Here's the drawing with two shaded views (mm, measured from the low corner). I have some questions. A direction names the side the tool comes from. Round coordinates to 2 decimals unless told otherwise and drop trailing zeros. Loops run counter-clockwise (first coordinate to the right, second up) from the corner with the lowest first, then second, coordinate; pieces in that order, holes last. Notation, with made-up numbers: (37.25, -3) -> (53.25, -3) arc R33 ccw to (53.25, 26) -> close; hole circle Ø7 at (53, -7). An arc over 180 degrees is marked (long way). Write item = value, one per line.
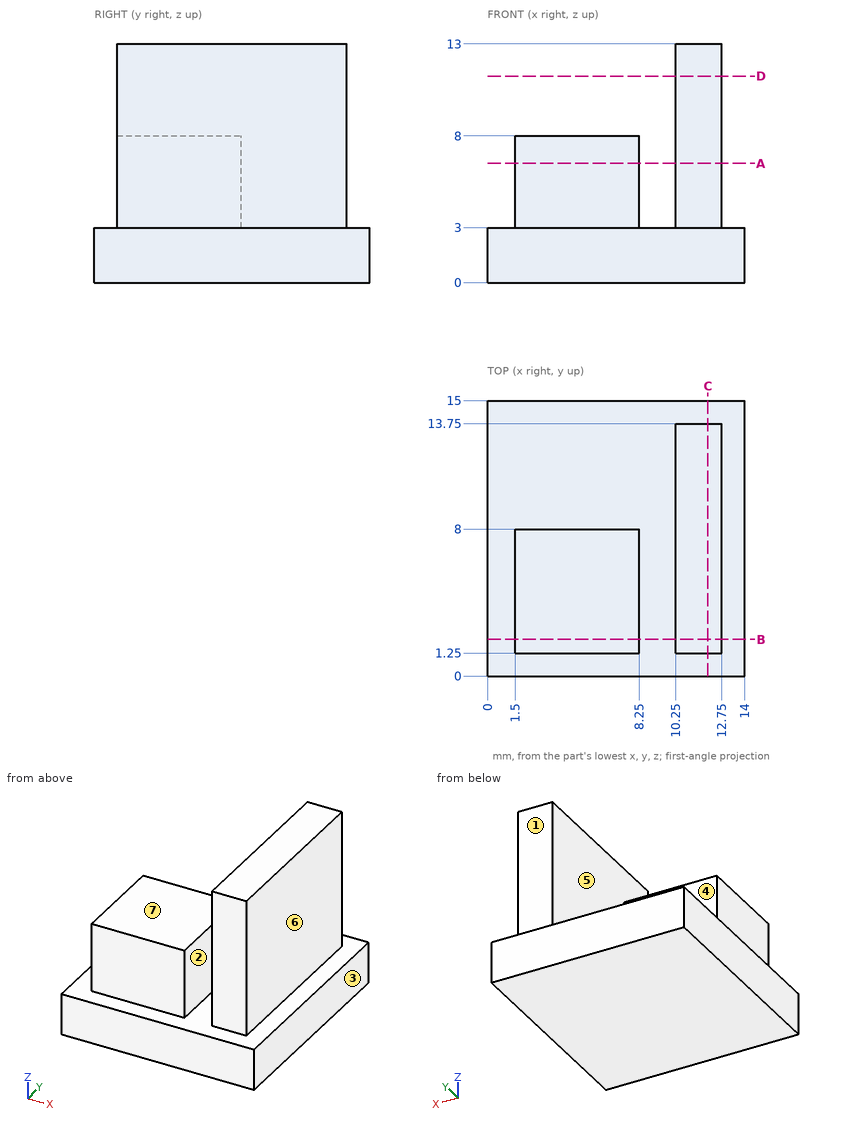
1. Suppose I cut it at C-C, the plane x = 12. List the corners of the cut face in (y, z) for me.
Entries:
outline = (0, 0) -> (15, 0) -> (15, 3) -> (13.75, 3) -> (13.75, 13) -> (1.25, 13) -> (1.25, 3) -> (0, 3) -> close
2. We'd pull the mould along X, two halves only. Please class the marked faces 1, 2 and 3: released by +X, released by -X, zero draft, split by the parting line, or undercut.
Entries:
face_1 = zero draft
face_2 = undercut
face_3 = released by +X
3. Suppose I cut it at A-A, the plane z = 6.5. List the corners of the cut face in (x, y) for me, and give its area (3 significant figures).
Entries:
outline = (1.5, 1.25) -> (8.25, 1.25) -> (8.25, 8) -> (1.5, 8) -> close; (10.25, 1.25) -> (12.75, 1.25) -> (12.75, 13.75) -> (10.25, 13.75) -> close
area = 76.8 mm²
4. For the marked faces 4, 5, 6 and 7, which set-ups out of +Z, -Z, +X, -X, +Y, -Y let a thin tool reach every point of the face, with its end or its side?
Entries:
face_4 = +Z, -X, +Y
face_5 = +Z, +Y, -Y
face_6 = +Z, +X, +Y, -Y
face_7 = +Z, -X, +Y, -Y
5. I need wall thicknesses on line 1 (X direction, y = 11, z = 7.5); line 2 (Z direction, x = 5.25, y = 6.25); line 3 (X direction, y = 5.75, z = 7.75). Which ranges of each line are inside material? Lowest first, please. Write a range as [from, to].
Entries:
line_1 = [10.25, 12.75]
line_2 = [0, 8]
line_3 = [1.5, 8.25], [10.25, 12.75]
6. Suppose I cut it at B-B, the plane y = 2. List the corners of the cut face in (x, z) for me.
Entries:
outline = (0, 0) -> (14, 0) -> (14, 3) -> (12.75, 3) -> (12.75, 13) -> (10.25, 13) -> (10.25, 3) -> (8.25, 3) -> (8.25, 8) -> (1.5, 8) -> (1.5, 3) -> (0, 3) -> close
7. Suppose I cut it at D-D, the plane z = 11.25. List the corners of the cut face in (x, y) for me.
Entries:
outline = (10.25, 1.25) -> (12.75, 1.25) -> (12.75, 13.75) -> (10.25, 13.75) -> close
8. I'm going to push flat-ended pins straight in: pin 1 (2.5 mm diameter, centred on y = 3, z = 6.5, fed in from +X); pin 2 (0.8 mm diameter, centred on x = 11.5, z = 9.5, fed in from -Y); pin 3 (1 mm diameter, centred on x = 2.5, z = 7.5, fed in from +Y). Where does each tip first touch, or does it pass through?
Entries:
pin_1 = 12.75
pin_2 = 1.25
pin_3 = 8
